Verification items for the finished model (mm, model axes). A direction names the side the tool comes from. Give positions to 0.01 mm unless a question says otherwise; leave off trailing zeros. Write each loop counter-clockwise with the first axis right and the second up, starting at its lowest first coordinate (ties: lowest second). Pieces come first, ordered by that corner, then holes. Notation, with made-up numbers: M 26,88 L 65,88 A7 cw 65,97 Z; hole C 47,34.5 d1. An arc over 180 degrees is marked long. Write item = value, one per line.
from build123d import *

# Parameters (mm, degrees)
F0_R     = 11.2
F1_DEPTH = 7


with BuildPart() as f1:
    # F0 (on Top) → F1 (new body)
    with BuildSketch(Plane.XY):
        with BuildLine():
            ThreePointArc((9.598043, 9.061875), (8.22906, 13.11739), (9.47712, 17.211736))
            ThreePointArc((9.47712, 17.211736), (9.935183, 17.801964), (10.453543, 18.34001))
            ThreePointArc((10.453543, 18.34001), (0, 39.6), (-10.453543, 18.34001))
            ThreePointArc((-10.453543, 18.34001), (-9.935183, 17.801964), (-9.47712, 17.211736))
            ThreePointArc((-9.47712, 17.211736), (-8.22906, 13.11739), (-9.598043, 9.061875))
            ThreePointArc((-9.598043, 9.061875), (-9.942486, 8.632092), (-10.319653, 8.230721))
            ThreePointArc((-10.319653, 8.230721), (-11.431535, 6.6), (-12.28784, 4.821721))
            ThreePointArc((-12.28784, 4.821721), (-12.446854, 4.294399), (-12.646835, 3.781212))
            ThreePointArc((-12.646835, 3.781212), (-15.474523, 0.56788), (-19.64436, -0.398441))
            ThreePointArc((-19.64436, -0.398441), (-20.384544, -0.296861), (-21.109686, -0.116971))
            ThreePointArc((-21.109686, -0.116971), (-34.294606, -19.8), (-10.656143, -18.223039))
            ThreePointArc((-10.656143, -18.223039), (-10.449362, -17.505103), (-10.16724, -16.813294))
            ThreePointArc((-10.16724, -16.813294), (-7.245463, -13.68527), (-3.048792, -12.843086))
            ThreePointArc((-3.048792, -12.843086), (-2.504368, -12.926492), (-1.968187, -13.052442))
            ThreePointArc((-1.968187, -13.052442), (0, -13.2), (1.968187, -13.052442))
            ThreePointArc((1.968187, -13.052442), (2.504368, -12.926492), (3.048792, -12.843086))
            ThreePointArc((3.048792, -12.843086), (7.245463, -13.68527), (10.16724, -16.813294))
            ThreePointArc((10.16724, -16.813294), (10.449362, -17.505103), (10.656143, -18.223039))
            ThreePointArc((10.656143, -18.223039), (34.294606, -19.8), (21.109686, -0.116971))
            ThreePointArc((21.109686, -0.116971), (20.384544, -0.296861), (19.64436, -0.398441))
            ThreePointArc((19.64436, -0.398441), (15.474523, 0.56788), (12.646835, 3.781212))
            ThreePointArc((12.646835, 3.781212), (12.446854, 4.294399), (12.28784, 4.821721))
            ThreePointArc((12.28784, 4.821721), (11.431535, 6.6), (10.319653, 8.230721))
            ThreePointArc((10.319653, 8.230721), (9.942486, 8.632092), (9.598043, 9.061875))
        make_face()
        with Locations((-22.863071, -13.2)):
            Circle(F0_R, mode=Mode.SUBTRACT)
        with Locations((22.863071, -13.2)):
            Circle(F0_R, mode=Mode.SUBTRACT)
        Circle(F0_R, mode=Mode.SUBTRACT)
        with Locations((0, 26.4)):
            Circle(F0_R, mode=Mode.SUBTRACT)
    extrude(amount=F1_DEPTH)


solid = f1.part
1) Cross-section at B-B on y = 26.4. Record the boundary of the cut face in (x, z).
From the geometry:
outline = M -13.2,0 L -11.2,0 L -11.2,7 L -13.2,7 Z; M 11.2,0 L 13.2,0 L 13.2,7 L 11.2,7 Z
2) Cross-section at A-A on x = 0. Record the boundary of the cut face in (y, z).
From the geometry:
outline = M -13.2,0 L -11.2,0 L -11.2,7 L -13.2,7 Z; M 11.2,0 L 15.2,0 L 15.2,7 L 11.2,7 Z; M 37.6,0 L 39.6,0 L 39.6,7 L 37.6,7 Z
3) Material ranges on probe 1 along Y at (x, z) = (0, 5.5); probe 2 along Y at (x, z) = (-23, 6.5); probe 3 along Y at (x, z) = (-5.5, 0.75), recorded low to high. Write a range as from..to.
From the geometry:
probe_1 = -13.2..-11.2, 11.2..15.2, 37.6..39.6
probe_2 = -26.4..-24.4, -2..0
probe_3 = -13..-9.76, 9.76..16.64, 36.16..38.4
4) Cross-section at C-C on z = 1. Record the boundary of the cut face in (x, y).
From the geometry:
outline = M -21.11,-0.12 A13.2 ccw long -10.66,-18.22 A7 cw -10.17,-16.81 A7 cw -3.05,-12.84 A7 cw -1.97,-13.05 A13.2 ccw 1.97,-13.05 A7 cw 3.05,-12.84 A7 cw 10.17,-16.81 A7 cw 10.66,-18.22 A13.2 ccw long 21.11,-0.12 A7 cw 12.65,3.78 A7 cw 12.29,4.82 A13.2 ccw 10.32,8.23 A7 cw 9.6,9.06 A7 cw 9.48,17.21 A7 cw 10.45,18.34 A13.2 ccw long -10.45,18.34 A7 cw -9.48,17.21 A7 cw -9.6,9.06 A7 cw -10.32,8.23 A13.2 ccw -12.29,4.82 A7 cw -12.65,3.78 A7 cw Z; hole C -22.86,-13.2 d22.4; hole C 0,0 d22.4; hole C 0,26.4 d22.4; hole C 22.86,-13.2 d22.4
5) Cross-section at D-D on x = 30. Record the boundary of the cut face in (y, z), plus the area to 3 significant figures.
From the geometry:
outline = M -24.3,0 L -21.83,0 L -21.83,7 L -24.3,7 Z; M -4.57,0 L -2.1,0 L -2.1,7 L -4.57,7 Z
area = 34.6 mm^2
6) Depth check by flat-ended pin: P1, Ø1.5, axis at y = 11, z = 0.5, coming from the -X side; P2, Ø1.5, axis at y = -1, z = 5.5, coming from the -X side; P3, Ø4, axis at x = 4, z = 4.5, coming from the +Y side; P4, Ø18, axis at x = 0, y = 0, coming from the +Z side. Enter the tip coordinate at first touch or a pass-through.
From the geometry:
P1 = -8.89
P2 = -29.43
P3 = 39.45
P4 = through
7) Tool access check on faces 5 (the cylindrical face through (-12.517, -17.49, 3.451)), 6 (the cylindrical face through (-11.42, 6.62, 3.45)). Record the directions out of +Z, -Z, +X, -X, +Y, -Y that give a thin tool (end or side, any length) a straight path to the whole face; none if there is none.
From the geometry:
face_5 = +Z, -Z
face_6 = +Z, -Z, -X
8) Draft check along Y on faces 1 (the cylindrical face through (0, -13.2, 3.5)), 2 (the cylindrical face through (34.083, -20.153, 3.451)), 3 (the cylindrical face through (11.445, 6.576, 3.451)), 4 (the flat face through (-8.2, -7.9, 0)). Enter one of: +Y half, -Y half, draft (parallel to the pull), parting line (faces both ways), or undercut.
From the geometry:
face_1 = -Y half
face_2 = parting line
face_3 = undercut
face_4 = draft
